Work out the finished part from the listing and answer in its coordinate system (mm). Face numbers are marked on the shaded views. A direction names the side the tool comes from. Round coordinates to 2 decimals unless told otherwise and drop trailing zeros. Answer in a Markdown table with one row per item.
```python
from build123d import *

# Parameters (mm, degrees)
SKETCH1_R                      = 115
BOSS_EXTRUDE1_DEPTH            = 40
CUT_EXTRUDE1_DEPTH             = 40
FILLET1_R                      = 6
SKETCH3_R                      = 4.25
CUT_EXTRUDE2_DEPTH             = 40
CIRPATTERN1_COUNT              = 7
FILLET1_OF_CIRPATTERN1_R       = 6
SKETCH4_R                      = 16
CUT_EXTRUDE3_DEPTH             = 5
M4_CLEARANCE_HOLE1_D           = 4.5
M4_CLEARANCE_HOLE1_DEPTH       = 13
M4_CLEARANCE_HOLE1_CSINK_D     = 4.55
M4_CLEARANCE_HOLE1_CSINK_ANGLE = 90
M4_CLEARANCE_HOLE1_TIP         = 1.351936393
FILLET2_R                      = 10


with BuildPart() as part:
    # Sketch1 → Boss-Extrude1 (new body)
    with BuildSketch(Plane(origin=(0, 0, 0), x_dir=(1, 0, 0), z_dir=(0, 1, 0))):
        Circle(SKETCH1_R)
    extrude(amount=BOSS_EXTRUDE1_DEPTH)

    # Sketch2 → Cut-Extrude1 (cut)
    with BuildSketch(Plane(origin=(0, 40, 0), x_dir=(1, 0, 0), z_dir=(0, 1, 0))):
        with BuildLine():
            ThreePointArc((-9.508910889, 20.391925208), (-4.869891314, 21.96666016), (0, 22.5))
            Line((0, 22.5), (0, 100))
            ThreePointArc((0, 100), (-21.643961394, 97.629600712), (-42.261826174, 90.630778704))
            Line((-42.261826174, 90.630778704), (-9.508910889, 20.391925208))
        make_face()
    cut_extrude1 = extrude(amount=-CUT_EXTRUDE1_DEPTH, mode=Mode.SUBTRACT)

    # Fillet1
    fillet1_edges = [part.edges().sort_by_distance(p)[0] for p in [
        (0, 20, -22.5),
        (-9.508910889, 20, -20.391925208),
        (-42.261826174, 20, -90.630778704),
        (0, 20, -100),
    ]]
    fillet(fillet1_edges, radius=FILLET1_R)

    # Sketch3 → Cut-Extrude2 (cut)
    with BuildSketch(Plane(origin=(0, 40, 0), x_dir=(1, 0, 0), z_dir=(0, 1, 0))):
        Circle(SKETCH3_R)
    extrude(amount=-CUT_EXTRUDE2_DEPTH, mode=Mode.SUBTRACT)

    # CirPattern1: Cut-Extrude1 ×7 about axis
    cirpattern1_axis = Axis((0, 0, 0), (0, 1, 0))
    for i in range(1, CIRPATTERN1_COUNT):
        add(cut_extrude1.rotate(cirpattern1_axis, i * 360 / CIRPATTERN1_COUNT), mode=Mode.SUBTRACT)

    # Fillet1 of CirPattern1
    fillet1_of_cirpattern1_edges = [part.edges().sort_by_distance(p)[0] for p in [
        (-17.591208356, 20, -14.028520542),
        (-21.871758082, 20, -5.279791511),
        (-97.207813699, 20, -23.465740047),
        (-78.183148247, 20, -62.348980186),
        (-21.935878024, 20, 5.006721014),
        (-17.764725337, 20, 13.808132883),
        (-78.95433483, 20, 61.369479479),
        (-97.492791218, 20, 22.252093396),
        (-9.76238413, 20, 20.271799528),
        (-0.280492078, 20, 22.498251581),
        (-1.24663146, 20, 99.992229248),
        (-43.388373912, 20, 90.09688679),
        (9.76238413, 20, 20.271799528),
        (17.414957436, 20, 14.246727958),
        (77.399810827, 20, 63.318790923),
        (43.388373912, 20, 90.09688679),
        (21.935878024, 20, 5.006721014),
        (21.996588801, 20, -4.732872398),
        (97.762616892, 20, -21.034988435),
        (97.492791218, 20, 22.252093396),
        (17.591208356, 20, -14.028520542),
        (10.01434015, 20, -20.148523305),
        (44.508178444, 20, -89.548992466),
        (78.183148247, 20, -62.348980186),
    ]]
    fillet(fillet1_of_cirpattern1_edges, radius=FILLET1_OF_CIRPATTERN1_R)

    # Sketch4 → Cut-Extrude3 (cut)
    with BuildSketch(Plane(origin=(0, 40, 0), x_dir=(1, 0, 0), z_dir=(0, 1, 0))):
        Circle(SKETCH4_R)
    extrude(amount=-CUT_EXTRUDE3_DEPTH, mode=Mode.SUBTRACT)

    # M4 Clearance Hole1
    with Locations(Plane(origin=(0, 35, 0), x_dir=(1, 0, 0), z_dir=(0, 1, 0))):
        with Locations((8, 8), (-8, 8), (-8, -8), (8, -8)):
            CounterSinkHole(M4_CLEARANCE_HOLE1_D / 2, M4_CLEARANCE_HOLE1_CSINK_D / 2, depth=M4_CLEARANCE_HOLE1_DEPTH, counter_sink_angle=M4_CLEARANCE_HOLE1_CSINK_ANGLE)
            with Locations((0, 0, -(M4_CLEARANCE_HOLE1_DEPTH + M4_CLEARANCE_HOLE1_TIP / 2))):  # 118° drill point
                Cone(0, M4_CLEARANCE_HOLE1_D / 2, M4_CLEARANCE_HOLE1_TIP, mode=Mode.SUBTRACT)

    # Fillet2
    fillet2_edges = [part.edges().sort_by_distance(p)[0] for p in [
        (-115, 0, 0),
        (-115, 40, 0),
    ]]
    fillet(fillet2_edges, radius=FILLET2_R)


solid = part.part
```
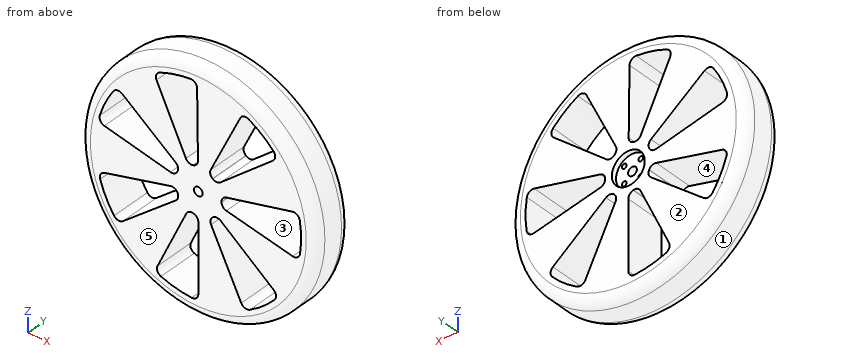
1. Consider line 1 along Z through (x, y) = (58.5, 38); line 2 along X through (y, z) = (14, -76.5); line 3 along X through (y, z) = (37, 85). Determine where each line is inside the solid, lowest interval first. Write a range as from..to.
Calculated:
| item | result |
|---|---|
| line 1 | z = -94.33..-81.1, -46.65..-12.59, 13.35..47.86, 81.1..94.33 |
| line 2 | x = -85.86..-35.67, 0..38.02, 64.4..85.86 |
| line 3 | x = -73.15..-40.91, -1.06..40.96, 52.68..73.15 |
2. Determine the mould class of the marked faces 1, 2 and 3 for opening direction X: released by +X, released by -X, zero draft, split by the parting line, or undercut.
Calculated:
| item | result |
|---|---|
| face 1 | split by the parting line |
| face 2 | zero draft |
| face 3 | undercut |
3. A tool of negligible diameter and unlimited length cuts with its end or side. For the marked faces 4 and 5, from which of +Z, -Z, +X, -X, +Y, -Y can it reach the whole face along a straight path? Write none if from no direction.
Calculated:
| item | result |
|---|---|
| face 4 | +Y, -Y |
| face 5 | +Z, -Z, +X, -X, -Y |
4. The part is cut by section A-A (y = 17). Count the separate pieces of the cut face and the enclosed holes in it, plus the area to 3 significant figures.
Calculated:
| item | result |
|---|---|
| separate pieces | 1 |
| enclosed holes | 8 |
| area | 27,200 mm² |
5. Given pin 1 (19 mm diameter, centred on x = 0, z = 0, fed in from +Y); pin 2 (4 mm diameter, centred on x = 8, z = -8, fed in from +Y); pin 3 (5 mm diameter, centred on y = 18, z = -29.5, fed in from +X), each flat-ended and moving along its own axis, determine where each tip first touches the part or whether it passes through.
Calculated:
| item | result |
|---|---|
| pin 1 | stops at y = 35 |
| pin 2 | stops at y = 21.85 |
| pin 3 | stops at x = 111.79 |
